Design review of the part built by this model. Coordinates are the model's own, in mm. Face numbers are marked on the shaded views. Give positions to 0.01 mm unless a question says otherwise; leave off trailing zeros. Loops run counter-clockwise (first coordinate to the right, second up) from the corner with the lowest first, then second, coordinate; pieces in that order, holes last. Notation, with made-up numbers: (39, 21.25) -> (45, 21.25) arc R21 ccw to (45, 57.25) -> close; hole circle Ø2 at (4, 4). An arc over 180 degrees is marked (long way). Answer in a Markdown table with one row per item. Add a question column.
(1) Consider section A-A on x = 0. Write out the cut boundary in (y, z), then the cut area to 3 significant figures.
(2) Draft analysis for pull direction X (two halves, no side actions). For the marked faces 1, 2 and 3, state which applies: +X half, -X half, draft (parallel to the pull), parting line (faces both ways), or undercut.
(3) Consider section D-D on y = -24. Write out the cut boundary in (x, z), then the cut area to 3 significant figures.
(4) For line 1 (Y direction, x = 0, z = 34); line 2 (Z direction, x = 18.5, y = 20.5); line 3 (Y direction, x = 0, z = -1.3), list the stretches that pass through material, from the lowest coordinate up.
(5) Consider section C-C on z = 23. Write out the cut boundary in (x, y).
(6) Consider section B-B on y = 16.96. Write out the cut boundary in (x, z).
(7) For pin 1 (3.5 mm diameter, centred on x = 0.5, y = -35.5, fed in from +Z); pin 2 (5 mm diameter, centred on y = -2, z = 9, fed in from +X); pin 3 (8 mm diameter, centred on y = -23.5, z = 35.5, fed in from -X); pin 4 (20 mm diameter, centred on x = 0, y = 16.96, fed in from +Z), all flat-tipped, find the tip position at first contact; note any pin that passes through.
from build123d import *

# Parameters (mm, degrees)
SKETCH1_R           = 37.5
SKETCH1_R_2         = 32.5
SKETCH1_R_3         = 31
BOSS_EXTRUDE1_DEPTH = 2
SKETCH2_R           = 32.5
SKETCH2_R_2         = 31
BOSS_EXTRUDE2_DEPTH = 55
SKETCH8_R           = 1.5
BOSS_EXTRUDE3_DEPTH = 10
CUT_EXTRUDE1_START  = -5
SKETCH9_R           = 32.5
SKETCH9_R_2         = 31
CUT_EXTRUDE1_DEPTH  = 5
SKETCH10_R          = 12.5
CUT_EXTRUDE3_DEPTH  = 100


with BuildPart() as part:
    # Sketch1 → Boss-Extrude1 (new body)
    # profile 1 of 3: a face of its own
    with BuildSketch(Plane.XY):
        Circle(SKETCH1_R)
        Circle(SKETCH1_R_2, mode=Mode.SUBTRACT)
    # profile 2 of 3: a face of its own
    with BuildSketch(Plane.XY):
        Circle(SKETCH1_R_2)
        Circle(SKETCH1_R_3, mode=Mode.SUBTRACT)
    # profile 3 of 3: a face of its own
    with BuildSketch(Plane.XY):
        Circle(SKETCH1_R_3)
    extrude(amount=-BOSS_EXTRUDE1_DEPTH)

    # Sketch2 → Boss-Extrude2 (add)
    with BuildSketch(Plane.XY):
        Circle(SKETCH2_R)
        Circle(SKETCH2_R_2, mode=Mode.SUBTRACT)
    extrude(amount=BOSS_EXTRUDE2_DEPTH)

    # Sketch8 → Boss-Extrude3 (add)
    with BuildSketch(Plane.XY):
        with Locations((0, 35)):
            Circle(SKETCH8_R)
        with Locations((0, -35)):
            Circle(SKETCH8_R)
    extrude(amount=BOSS_EXTRUDE3_DEPTH)

    # Sketch9 → Cut-Extrude1 (cut)
    with BuildSketch(Plane.XY.offset(55).offset(CUT_EXTRUDE1_START)):
        Circle(SKETCH9_R)
        Circle(SKETCH9_R_2, mode=Mode.SUBTRACT)
    extrude(amount=CUT_EXTRUDE1_DEPTH, mode=Mode.SUBTRACT)

    # Sketch10 → Cut-Extrude3 (cut)
    with BuildSketch(Plane(origin=(0, 0, -2), x_dir=(-1, 0, 0), z_dir=(0, 0, -1))):
        with Locations((0, 16.96)):
            Circle(SKETCH10_R)
    extrude(amount=-CUT_EXTRUDE3_DEPTH, mode=Mode.SUBTRACT)


solid = part.part
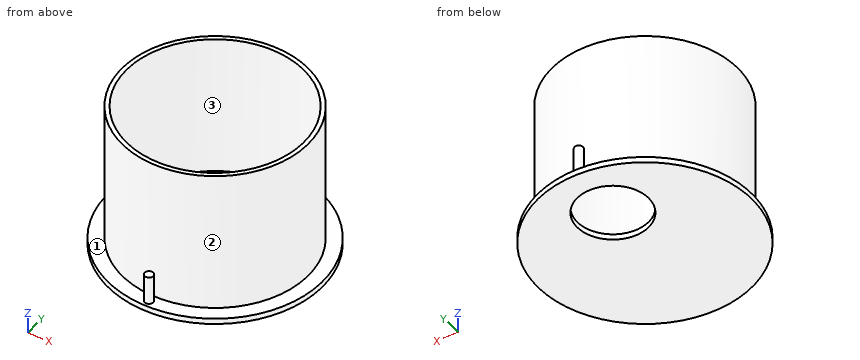
Values follow:
| question | item | result |
|---|---|---|
| 1 | outline | (-37.5, -2) -> (4.46, -2) -> (4.46, 0) -> (-31, 0) -> (-31, 50) -> (-32.5, 50) -> (-32.5, 0) -> (-33.5, 0) -> (-33.5, 10) -> (-36.5, 10) -> (-36.5, 0) -> (-37.5, 0) -> close; (29.46, -2) -> (37.5, -2) -> (37.5, 0) -> (36.5, 0) -> (36.5, 10) -> (33.5, 10) -> (33.5, 0) -> (32.5, 0) -> (32.5, 50) -> (31, 50) -> (31, 0) -> (29.46, 0) -> close |
| 1 | area | 310 mm2 |
| 2 | face 1 | draft |
| 2 | face 2 | parting line |
| 2 | face 3 | undercut |
| 3 | outline | (-28.81, -2) -> (28.81, -2) -> (28.81, 0) -> (21.91, 0) -> (21.91, 50) -> (19.62, 50) -> (19.62, 0) -> (-19.62, 0) -> (-19.62, 50) -> (-21.91, 50) -> (-21.91, 0) -> (-28.81, 0) -> close |
| 3 | area | 345 mm2 |
| 4 | line 1 | -32.5 to -31, 31 to 32.5 |
| 4 | line 2 | -2 to 0 |
| 4 | line 3 | -37.5 to 4.46, 29.46 to 37.5 |
| 5 | outline | circle Ø65 at (0, 0); hole circle Ø62 at (0, 0) |
| 6 | outline | (-33.45, -2) -> (-12.5, -2) -> (-12.5, 0) -> (-25.95, 0) -> (-25.95, 50) -> (-27.72, 50) -> (-27.72, 0) -> (-33.45, 0) -> close; (12.5, -2) -> (33.45, -2) -> (33.45, 0) -> (27.72, 0) -> (27.72, 50) -> (25.95, 50) -> (25.95, 0) -> (12.5, 0) -> close |
| 7 | pin 1 | z = 10 |
| 7 | pin 2 | x = 32.5 |
| 7 | pin 3 | x = -26 |
| 7 | pin 4 | through |
